from build123d import *

# Parameters (mm, degrees)
EXTRUDE_1_DEPTH     = 5
SKETCH_3_R          = 1.25
CUT_EXTRUDE_2_DEPTH = 7.5
SKETCH_4_R          = 1.25
CUT_EXTRUDE_3_DEPTH = 76.013332148
SKETCH_5_R          = 0.75
CUT_EXTRUDE_4_DEPTH = 76.013332148
SKETCH_6_R          = 1.5
CUT_EXTRUDE_5_DEPTH = 76.013332148


with BuildPart() as part:
    # ｽｹｯﾁ1 → ﾎﾞｽ - 押し出し1 (new body)
    with BuildSketch(Plane.XY):
        Polygon((-29, 51), (-29, 0), (-23, 0), (-23, -3), (23, -3), (23, 0), (29, 0), (29, 51), (23, 51), (23, 69), (-23, 69), (-23, 51), align=None)
    extrude(amount=EXTRUDE_1_DEPTH)

    # ｽｹｯﾁ3 → ｶｯﾄ - 押し出し2 (cut)
    with BuildSketch(Plane(origin=(0, 51, 0), x_dir=(1, 0, 0), z_dir=(0, 1, 0))):
        with Locations(Location((-26, -2.5, 0), (0, 0, 270))):
            Circle(SKETCH_3_R)
        with Locations(Location((26, -2.5, 0), (0, 0, 270))):
            Circle(SKETCH_3_R)
    cut_extrude_2 = extrude(amount=-CUT_EXTRUDE_2_DEPTH, mode=Mode.SUBTRACT)

    # ﾐﾗｰ1: ｶｯﾄ - 押し出し2 across plane
    add(cut_extrude_2.mirror(Plane.ZX.offset(25.5)), mode=Mode.SUBTRACT)

    # ｽｹｯﾁ4 → ｶｯﾄ - 押し出し3 (cut, through all)
    with BuildSketch(Plane(origin=(0, 0, 0), x_dir=(-1, 0, 0), z_dir=(0, 0, -1))):
        with Locations((-20.5, 66.5)):
            Circle(SKETCH_4_R)
        with Locations((20.5, 66.5)):
            Circle(SKETCH_4_R)
    extrude(amount=-CUT_EXTRUDE_3_DEPTH, mode=Mode.SUBTRACT)

    # ｽｹｯﾁ5 → ｶｯﾄ - 押し出し4 (cut, through all)
    with BuildSketch(Plane(origin=(0, 0, 0), x_dir=(-1, 0, 0), z_dir=(0, 0, -1))):
        with Locations((-23, 0)):
            Circle(SKETCH_5_R)
        with Locations((23, 0)):
            Circle(SKETCH_5_R)
        with Locations((-23, 51)):
            Circle(SKETCH_5_R)
        with Locations((23, 51)):
            Circle(SKETCH_5_R)
    extrude(amount=-CUT_EXTRUDE_4_DEPTH, mode=Mode.SUBTRACT)

    # ｽｹｯﾁ6 → ｶｯﾄ - 押し出し5 (cut, through all)
    with BuildSketch(Plane(origin=(0, 0, 0), x_dir=(-1, 0, 0), z_dir=(0, 0, -1))):
        with Locations((-26, 44)):
            Circle(SKETCH_6_R)
        with Locations(Location((-26, 7, 0), (0, 0, 180))):
            Circle(SKETCH_6_R)
        with Locations((26, 7)):
            Circle(SKETCH_6_R)
        with Locations(Location((26, 44, 0), (0, 0, 180))):
            Circle(SKETCH_6_R)
    extrude(amount=-CUT_EXTRUDE_5_DEPTH, mode=Mode.SUBTRACT)


solid = part.part
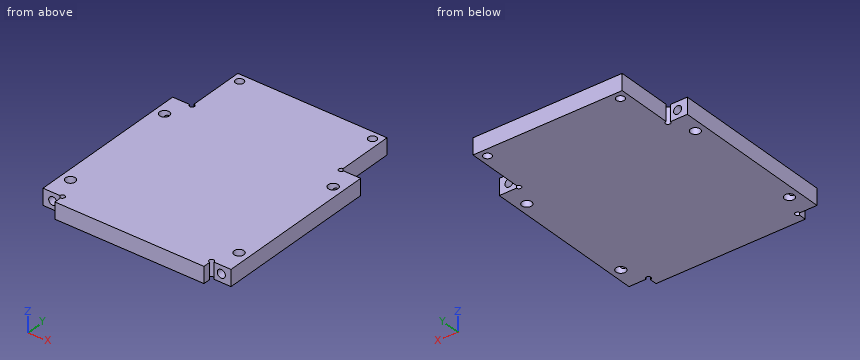
The model under review builds one solid part; all positions refer to its coordinate system, in mm. Round coordinates to 2 decimals unless told otherwise and drop trailing zeros. Loops run counter-clockwise (first coordinate to the right, second up) from the corner with the lowest first, then second, coordinate; pieces in that order, holes last. Notation, with made-up numbers: (-17, -15) -> (36, -15) arc R7 cw to (36, -8) -> close; hole circle Ø11 at (-2.75, 36). An arc over 180 degrees is marked (long way). Return JSON: item names as keys, results as strings.
(1) Add section D-D on y = 66.5. Write out the cut boundary in (x, z), plus the area to 3 significant figures.
Solved:
{"outline": "(-23, 0) -> (-21.75, 0) -> (-21.75, 5) -> (-23, 5) -> close; (-19.25, 0) -> (19.25, 0) -> (19.25, 5) -> (-19.25, 5) -> close; (21.75, 0) -> (23, 0) -> (23, 5) -> (21.75, 5) -> close", "area": "205 mm2"}
(2) For line 1 (X direction, y = 47.5, z = 2.5); line 2 (Y direction, x = 26, z = 4.6); line 3 (Z direction, x = -26, y = 48.5), list the stretches that pass through material, from the lowest coordinate up.
Solved:
{"line 1": "-29 to -27.25, -24.75 to 24.75, 27.25 to 29", "line 2": "0 to 5.5, 8.5 to 42.5, 45.5 to 51", "line 3": "0 to 1.25, 3.75 to 5"}
(3) Add section A-A on x = -26. Write out the cut boundary in (y, z), plus the area to 4 significant figures.
Solved:
{"outline": "(0, 0) -> (5.5, 0) -> (5.5, 1.25) -> (0, 1.25) -> close; (0, 3.75) -> (5.5, 3.75) -> (5.5, 5) -> (0, 5) -> close; (8.5, 0) -> (42.5, 0) -> (42.5, 5) -> (8.5, 5) -> close; (45.5, 0) -> (51, 0) -> (51, 1.25) -> (45.5, 1.25) -> close; (45.5, 3.75) -> (51, 3.75) -> (51, 5) -> (45.5, 5) -> close", "area": "197.5 mm2"}
(4) For pin 1 (2.5 mm diameter, centred on x = 27, z = 3.5, fed in from -Y); pin 2 (2.5 mm diameter, centred on y = -2, z = 3.5, fed in from +X); pin 3 (2 mm diameter, centred on x = -26, z = 2.5, fed in from +Y), all flat-tipped, find the tip position at first contact; note any pin that passes through.
Solved:
{"pin 1": "y = 0", "pin 2": "x = 23", "pin 3": "y = 42.88"}
(5) Add section C-C on y = 7. Write out the cut boundary in (x, z).
Solved:
{"outline": "(-29, 0) -> (-27.5, 0) -> (-27.5, 5) -> (-29, 5) -> close; (-24.5, 0) -> (24.5, 0) -> (24.5, 5) -> (-24.5, 5) -> close; (27.5, 0) -> (29, 0) -> (29, 5) -> (27.5, 5) -> close"}
(6) Add section B-B on z = 2.5. State how many separate pieces and enclosed holes the cut face has, plus the area to 3 significant figures.
Solved:
{"separate pieces": "1", "enclosed holes": "2", "area": "3,820 mm2"}
